Here's how the part is built. I have some questions about the finished solid (model axes, mm). A direction names the side the tool comes from. Round coordinates to 2 decimals unless told otherwise and drop trailing zeros. Write each loop counter-clockwise with the first axis right and the second up, starting at its lowest first coordinate (ties: lowest second). Pieces come first, ordered by that corner, then holes. Notation, with made-up numbers: (-30.75, -17.5) - (25.25, -17.5) arc R9 cw to (25.25, -12.5) - close; hole circle Ø6 at (6, 9). An arc over 180 degrees is marked (long way). Use one line per item in the form item = value. Start each with the question number.
1. I want a section at A-A, the plane z = 2. List the corners of the cut face in (x, y) for me, plus the area to 3 significant figures.
2. Will this pin go through, and if not, where does the flat tip stop? pin 1 (1.2 mm diameter, centred on x = 9, z = -6, fed in from -Y).
3. We'd pull the mould along Y, two halves only. Please class faces 1 (the flat face through (12.7, -1, 0)), 2 (the flat face through (0, 0, 0)), 3 (the flat face through (9, -1.27, -6)): +Y half, -Y half, draft (parallel to the pull), parting line (faces both ways), or undercut.
4. Which directions (+Z, -Z, +X, -X, +Y, -Y) give clear straight access to the entire face, cutting with the end or side of a thin tool? Please do faces 4 (the flat face through (-9, -1.27, -6)), 5 (the cylindrical face through (11.936, -0.644, 19.596)).
5. If I drill on line 1 along Y through (x, z) = (7.75, -14.5); line 2 along Z through (x, y) = (11.5, -0.1); line 3 along Z through (x, y) = (11, -1), over which ranges is the centre line in solid material (lowest first)?
6. I want a section at B-B, the plane x = -9.25. List the corners of the cut face in (y, z) for me, plus the area to 3 significant figures.
```python
from build123d import *

# Parameters (mm, degrees)
F0_W     = 25.4
F0_H     = 40.64
F1_DEPTH = 1.27
F2_R     = 2.032
F3_DEPTH = 0.254
F4_R     = 2.54
F5_R     = 1.27


# Not quite as in the source:
# - the dataset's text gives a spline's control points without its knots; the knots are read off the source's solid


with BuildPart() as f1:
    # F0 (on Front) → F1 (new body)
    with BuildSketch(Plane.XZ):
        Rectangle(F0_W, F0_H)
    extrude(amount=F1_DEPTH)

    # F2 (on face) → F3 (join)
    with BuildSketch(Plane.XZ.offset(1.27)):
        with BuildLine():
            ThreePointArc((-7.5180080999, -7.4846331009), (-6.8898600985, -6.6273003834), (-6.6675, -5.588))
            ThreePointArc((-6.6675, -5.588), (-9.0473495717, -3.0530538782), (-11.7273045987, -5.268336451))
            ThreePointArc((-11.7273045987, -5.268336451), (-10.3908627949, -7.8354991648), (-7.5180080999, -7.4846331009))
        make_face()
        with Locations((-9.2075, -5.588)):
            Circle(F2_R, mode=Mode.SUBTRACT)
        with BuildLine():
            ThreePointArc((-11.7273045987, -5.268336451), (-9.0473495717, -3.0530538782), (-6.6675, -5.588))
            ThreePointArc((-6.6675, -5.588), (-6.8898600985, -6.6273003834), (-7.5180080999, -7.4846331009))
            add(Edge.make_bspline(
                [(-1.4182194217, -5.4769095653), (-4.1012740694, -5.0478749908), (-5.7548377663, -5.9140278026), (-7.5180080999, -7.4846331009)],
                knots=[0, 0, 0, 0, 6.4217112762, 6.4217112762, 6.4217112762, 6.4217112762], degree=3))
            add(Edge.make_bspline(
                [(-5.08, -2.794), (-5.08, -4.8913715579), (-1.4182194217, -5.4769095653)],
                knots=[3.1415926536, 3.1415926536, 3.1415926536, 4.4294520022, 4.4294520022, 4.4294520022], degree=2, weights=[1, 0.7997427872, 1]))
            add(Edge.make_bspline(
                [(5.08, -2.794), (5.08, 0), (0, 0), (-5.08, 0), (-5.08, -2.794)],
                knots=[0, 0, 0, 1.5707963268, 1.5707963268, 3.1415926536, 3.1415926536, 3.1415926536], degree=2, weights=[1, 0.7071067812, 1, 0.7071067812, 1]))
            add(Edge.make_bspline(
                [(1.4182194217, -5.4769095653), (5.08, -4.8913715579), (5.08, -2.794)],
                knots=[4.9953259586, 4.9953259586, 4.9953259586, 6.2831853072, 6.2831853072, 6.2831853072], degree=2, weights=[1, 0.7997427872, 1]))
            add(Edge.make_bspline(
                [(1.4182194217, -5.4769095653), (4.1012740694, -5.0478749908), (5.7548377663, -5.9140278026), (7.5180080999, -7.4846331009)],
                knots=[0, 0, 0, 0, 6.4217112762, 6.4217112762, 6.4217112762, 6.4217112762], degree=3))
            ThreePointArc((7.5180080999, -7.4846331009), (8.0241372051, -3.3405008352), (11.7273045987, -5.268336451))
            add(Edge.make_bspline(
                [(11.43, -2.9357403982), (11.43, -3.7171181073), (11.6289668146, -4.4931714335), (11.7273045987, -5.268336451)],
                knots=[0, 0, 0, 0, 2.3514664297, 2.3514664297, 2.3514664297, 2.3514664297], degree=3))
            Line((11.43, -2.9357403982), (11.43, 19.05))
            Line((11.43, 19.05), (-11.43, 19.05))
            Line((-11.43, 19.05), (-11.43, -2.9357403982))
            add(Edge.make_bspline(
                [(-11.43, -2.9357403982), (-11.43, -3.7171181073), (-11.6289668146, -4.4931714335), (-11.7273045987, -5.268336451)],
                knots=[0, 0, 0, 0, 2.3514664297, 2.3514664297, 2.3514664297, 2.3514664297], degree=3))
        make_face()
        with BuildLine():
            add(Edge.make_bspline(
                [(-5.08, -2.794), (-5.08, -4.8913715579), (-1.4182194217, -5.4769095653)],
                knots=[3.1415926536, 3.1415926536, 3.1415926536, 4.4294520022, 4.4294520022, 4.4294520022], degree=2, weights=[1, 0.7997427872, 1]))
            add(Edge.make_bspline(
                [(-1.4182194217, -5.4769095653), (0, -5.7036903231), (1.4182194217, -5.4769095653)],
                knots=[4.4294520022, 4.4294520022, 4.4294520022, 4.9953259586, 4.9953259586, 4.9953259586], degree=2, weights=[1, 0.960239644, 1]))
            add(Edge.make_bspline(
                [(1.4182194217, -5.4769095653), (5.08, -4.8913715579), (5.08, -2.794)],
                knots=[4.9953259586, 4.9953259586, 4.9953259586, 6.2831853072, 6.2831853072, 6.2831853072], degree=2, weights=[1, 0.7997427872, 1]))
            add(Edge.make_bspline(
                [(5.08, -2.794), (5.08, 0), (0, 0), (-5.08, 0), (-5.08, -2.794)],
                knots=[0, 0, 0, 1.5707963268, 1.5707963268, 3.1415926536, 3.1415926536, 3.1415926536], degree=2, weights=[1, 0.7071067812, 1, 0.7071067812, 1]))
        make_face()
        with BuildLine():
            add(Edge.make_bspline(
                [(-4.572, -2.794), (-4.572, -2.9169028513), (-4.5290705478, -3.1627085538), (-4.3175460933, -3.5550013791), (-3.9283471819, -3.9595979757), (-3.3716681218, -4.3337764728), (-2.6686840163, -4.6525156626), (-1.8416721788, -4.8959053951), (-0.9445084224, -5.0455757275), (0, -5.0972121363), (0.9445084224, -5.0455757275), (1.8416721788, -4.8959053951), (2.6686840163, -4.6525156626), (3.3716681218, -4.3337764728), (3.9283471819, -3.9595979757), (4.3175460933, -3.5550013791), (4.5290705478, -3.1627085538), (4.5934647261, -2.794), (4.5290705478, -2.4252914462), (4.3175460933, -2.0329986209), (3.9283471819, -1.6284020243), (3.3716681218, -1.2542235272), (2.6686840163, -0.9354843374), (1.8416721788, -0.6920946049), (0.9445084224, -0.5424242725), (0, -0.4907878637), (-0.9445084224, -0.5424242725), (-1.8416721788, -0.6920946049), (-2.6686840163, -0.9354843374), (-3.3716681218, -1.2542235272), (-3.9283471819, -1.6284020243), (-4.3175460933, -2.0329986209), (-4.5290705478, -2.4252914462), (-4.572, -2.6710971487), (-4.572, -2.794)],
                knots=[0, 0, 0, 0, 0.03125, 0.0625, 0.09375, 0.125, 0.15625, 0.1875, 0.21875, 0.25, 0.28125, 0.3125, 0.34375, 0.375, 0.40625, 0.4375, 0.46875, 0.5, 0.53125, 0.5625, 0.59375, 0.625, 0.65625, 0.6875, 0.71875, 0.75, 0.78125, 0.8125, 0.84375, 0.875, 0.90625, 0.9375, 0.96875, 1, 1, 1, 1], degree=3))
        make_face(mode=Mode.SUBTRACT)
        with BuildLine():
            ThreePointArc((11.7273045987, -5.268336451), (8.0241372051, -3.3405008352), (7.5180080999, -7.4846331009))
            ThreePointArc((7.5180080999, -7.4846331009), (10.2468003834, -7.9056399015), (11.7475, -5.588))
            ThreePointArc((11.7475, -5.588), (11.7424461218, -5.4278495717), (11.7273045987, -5.268336451))
        make_face()
        with Locations((9.2075, -5.588)):
            Circle(F2_R, mode=Mode.SUBTRACT)
    extrude(amount=F3_DEPTH)

    # F4
    f4_edges = [f1.edges().sort_by_distance(p)[0] for p in [
        (12.7, -0.635, -20.32),
        (-12.7, -0.635, -20.32),
        (-12.7, -0.635, 20.32),
        (12.7, -0.635, 20.32),
    ]]
    fillet(f4_edges, radius=F4_R)

    # F5
    f5_edges = [f1.edges().sort_by_distance(p)[0] for p in [
        (-11.43, -1.397, 19.05),
        (11.43, -1.397, 19.05),
    ]]
    fillet(f5_edges, radius=F5_R)


solid = f1.part
```
Model answer:
q1.outline = (-12.7, -1.27) - (-11.43, -1.27) - (-11.43, -1.52) - (11.43, -1.52) - (11.43, -1.27) - (12.7, -1.27) - (12.7, 0) - (-12.7, 0) - close
q1.area = 38.1 mm2
q2.pin_1 = -1.27
q3.face_1 = draft
q3.face_2 = +Y half
q3.face_3 = -Y half
q4.face_4 = -Y
q4.face_5 = +Z, +X, +Y, -Y
q5.line_1 = -1.27 to 0
q5.line_2 = -19.94 to 19.94
q5.line_3 = -20.18 to 20.18
q6.outline = (-1.52, -8.13) - (-1.27, -8.13) - (-1.27, -20.32) - (0, -20.32) - (0, 20.32) - (-1.27, 20.32) - (-1.27, 19.05) - (-1.52, 19.05) - (-1.52, -3.56) - (-1.27, -3.56) - (-1.27, -7.62) - (-1.52, -7.62) - close
q6.area = 57.5 mm2
